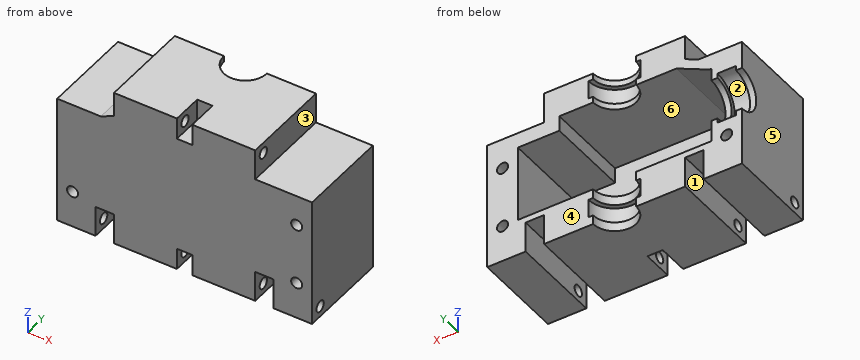
```python
from build123d import *

# Parameters (mm, degrees)
BOSS_EXTRUDE1_DEPTH  = 30
CUT_EXTRUDE2_START   = 2.5
CUT_EXTRUDE2_DEPTH   = 27.5
CUT_EXTRUDE3_START   = -2
SKETCH3_R            = 8.5
CUT_EXTRUDE3_DEPTH   = 6
CUT_EXTRUDE4_START   = -9
SKETCH4_R            = 8.5
CUT_EXTRUDE4_DEPTH   = 6
CUT_EXTRUDE6_DEPTH   = 73.981161953
SKETCH16_W           = 6
SKETCH16_H           = 30
CUT_EXTRUDE7_DEPTH   = 10
CUT_EXTRUDE8_START   = 2
SKETCH17_R           = 8.5
CUT_EXTRUDE8_DEPTH   = 6
CUT_EXTRUDE9_REACH   = 98.897
CHAMFER1_SIZE        = 2
CHAMFER1_SIZE2       = 4.289013841
CHAMFER2_SIZE        = 12.867041523
CHAMFER2_SIZE_2      = 6
SKETCH19_W           = 5
SKETCH19_H           = 7
CUT_EXTRUDE11_DEPTH  = 10
M3_CLEARANCE_HOLE1_D = 3.6
M3_CLEARANCE_HOLE2_D = 3.6


with BuildPart() as part:
    # Sketch1 → Boss-Extrude1 (new body)
    with BuildSketch(Plane(origin=(0, 0, 0), x_dir=(1, 0, 0), z_dir=(0, 1, 0))):
        Polygon((-41.5, 12), (41.5, 12), (41.5, -15), (41.5, -30), (23, -30), (23, -40), (-23, -40), (-23, -30), (-41.5, -30), (-41.5, -15), align=None)
    extrude(amount=BOSS_EXTRUDE1_DEPTH)

    # Sketch1<4> → Cut-Extrude2 (cut)
    with BuildSketch(Plane(origin=(0, 0, 0), x_dir=(1, 0, 0), z_dir=(0, 1, 0)).offset(CUT_EXTRUDE2_START)):
        Polygon((31.5, 0), (-31.5, 0), (-31.5, -10), (-31.5, -25), (-18, -25), (-18, -30), (18, -30), (18, -25), (31.5, -25), (31.5, -10), align=None)
    extrude(amount=CUT_EXTRUDE2_DEPTH, mode=Mode.SUBTRACT)

    # Sketch3 → Cut-Extrude3 (cut)
    with BuildSketch(Plane.XY.offset(40).offset(CUT_EXTRUDE3_START)):
        with Locations((0, 30)):
            Circle(SKETCH3_R)
    extrude(amount=-CUT_EXTRUDE3_DEPTH, mode=Mode.SUBTRACT)

    # Sketch4 → Cut-Extrude4 (cut)
    with BuildSketch(Plane(origin=(0, 0, -12), x_dir=(-1, 0, 0), z_dir=(0, 0, -1)).offset(CUT_EXTRUDE4_START)):
        with Locations((0, 30)):
            Circle(SKETCH4_R)
    extrude(amount=CUT_EXTRUDE4_DEPTH, mode=Mode.SUBTRACT)

    # Sketch3<4> → Cut-Extrude6 (cut, through all)
    with BuildSketch(Plane.XY.offset(40)):
        with BuildLine():
            Line((-7, 30), (7, 30))
            ThreePointArc((7, 30), (0, 37), (-7, 30))
        make_face()
        with BuildLine():
            ThreePointArc((-7, 30), (0, 23), (7, 30))
            Line((7, 30), (-7, 30))
        make_face()
        with BuildLine():
            Line((-7, 30), (7, 30))
            ThreePointArc((7, 30), (0, 37), (-7, 30))
        make_face()
        with BuildLine():
            ThreePointArc((-7, 30), (0, 23), (7, 30))
            Line((7, 30), (-7, 30))
        make_face()
    extrude(amount=-CUT_EXTRUDE6_DEPTH, mode=Mode.SUBTRACT)

    # Sketch16 → Cut-Extrude7 (cut)
    with BuildSketch(Plane(origin=(0, 0, -12), x_dir=(-1, 0, 0), z_dir=(0, 0, -1))):
        with Locations((26, 15)):
            Rectangle(SKETCH16_W, SKETCH16_H)
        with Locations((-26, 15)):
            Rectangle(SKETCH16_W, SKETCH16_H)
    extrude(amount=-CUT_EXTRUDE7_DEPTH, mode=Mode.SUBTRACT)

    # Sketch17 → Cut-Extrude8 (cut)
    with BuildSketch(Plane(origin=(-41.5, 0, 0), x_dir=(0, 0, -1), z_dir=(1, 0, 0)).offset(CUT_EXTRUDE8_START)):
        with Locations((-14, 30)):
            Circle(SKETCH17_R)
    extrude(amount=CUT_EXTRUDE8_DEPTH, mode=Mode.SUBTRACT)

    # Cut-Extrude9: up to this face of the body (flat: up to its plane)
    cut_extrude9_end = Plane(part.part.faces().sort_by_distance((-31.5, 16.25, 12.5))[0])
    # Sketch17<3> → Cut-Extrude9 (cut, up to the picked face)
    with BuildSketch(Plane(origin=(-41.5, 0, 0), x_dir=(0, 0, -1), z_dir=(1, 0, 0)), mode=Mode.PRIVATE) as cut_extrude9_sk1:
        with BuildLine():
            Line((-21, 30), (-7, 30))
            ThreePointArc((-7, 30), (-14, 37), (-21, 30))
        make_face()
    cut_extrude9_tool1 = split(extrude(cut_extrude9_sk1.sketch, amount=CUT_EXTRUDE9_REACH, mode=Mode.PRIVATE), bisect_by=cut_extrude9_end, keep=Keep.BOTH, mode=Mode.PRIVATE)
    # Sketch17<3> → Cut-Extrude9 (cut, up to the picked face)
    with BuildSketch(Plane(origin=(-41.5, 0, 0), x_dir=(0, 0, -1), z_dir=(1, 0, 0)), mode=Mode.PRIVATE) as cut_extrude9_sk2:
        with BuildLine():
            ThreePointArc((-21, 30), (-14, 23), (-7, 30))
            Line((-7, 30), (-21, 30))
        make_face()
    cut_extrude9_tool2 = split(extrude(cut_extrude9_sk2.sketch, amount=CUT_EXTRUDE9_REACH, mode=Mode.PRIVATE), bisect_by=cut_extrude9_end, keep=Keep.BOTH, mode=Mode.PRIVATE)
    # Sketch17<3> → Cut-Extrude9 (cut, up to the picked face)
    with BuildSketch(Plane(origin=(-41.5, 0, 0), x_dir=(0, 0, -1), z_dir=(1, 0, 0)), mode=Mode.PRIVATE) as cut_extrude9_sk3:
        with BuildLine():
            Line((-21, 30), (-7, 30))
            ThreePointArc((-7, 30), (-14, 37), (-21, 30))
        make_face()
    cut_extrude9_tool3 = split(extrude(cut_extrude9_sk3.sketch, amount=CUT_EXTRUDE9_REACH, mode=Mode.PRIVATE), bisect_by=cut_extrude9_end, keep=Keep.BOTH, mode=Mode.PRIVATE)
    # Sketch17<3> → Cut-Extrude9 (cut, up to the picked face)
    with BuildSketch(Plane(origin=(-41.5, 0, 0), x_dir=(0, 0, -1), z_dir=(1, 0, 0)), mode=Mode.PRIVATE) as cut_extrude9_sk4:
        with BuildLine():
            ThreePointArc((-21, 30), (-14, 23), (-7, 30))
            Line((-7, 30), (-21, 30))
        make_face()
    cut_extrude9_tool4 = split(extrude(cut_extrude9_sk4.sketch, amount=CUT_EXTRUDE9_REACH, mode=Mode.PRIVATE), bisect_by=cut_extrude9_end, keep=Keep.BOTH, mode=Mode.PRIVATE)
    add(cut_extrude9_tool1.solids().sort_by(Axis((-41.5, 32.970892, 14), (1, 0, 0)))[0], mode=Mode.SUBTRACT)
    add(cut_extrude9_tool2.solids().sort_by(Axis((-41.5, 27.029108, 14), (1, 0, 0)))[0], mode=Mode.SUBTRACT)
    add(cut_extrude9_tool3.solids().sort_by(Axis((-41.5, 32.970892, 14), (1, 0, 0)))[0], mode=Mode.SUBTRACT)
    add(cut_extrude9_tool4.solids().sort_by(Axis((-41.5, 27.029108, 14), (1, 0, 0)))[0], mode=Mode.SUBTRACT)

    # Chamfer1
    chamfer1_edges = [part.edges().sort_by_distance(p)[0] for p in [
        (-23, 15, 30),
    ]]
    chamfer1_side = [part.faces().sort_by_distance(p)[0] for p in [
        (-23, 15, 35),
    ]]
    chamfer(chamfer1_edges, length=CHAMFER1_SIZE, length2=CHAMFER1_SIZE2, reference=chamfer1_side[0])

    # Chamfer2
    # the kernel refuses this chamfer: 12.867041523, 6 mm, written as the material it takes off along each edge
    with BuildSketch(Plane(origin=(-18, 2.5, 25), x_dir=(-0.9998669641130704, 0, -0.016311164131110355), z_dir=(0, 1, 0))) as chamfer2_piece_1_section:
        Polygon((CHAMFER2_SIZE * 0.999866964118, CHAMFER2_SIZE * 0.0163111641312), (-CHAMFER2_SIZE_2 * 0.0163111641311, CHAMFER2_SIZE_2 * 0.999866964113), (0, 0), align=None)
    chamfer2_piece_1 = extrude(amount=60.838188976, mode=Mode.PRIVATE)
    chamfer2_piece_1 = split(chamfer2_piece_1, bisect_by=Plane(origin=(-22.391133218, 16.25, 30), z_dir=(0, 0, -1)), keep=Keep.TOP, mode=Mode.PRIVATE)
    add(chamfer2_piece_1, mode=Mode.SUBTRACT)

    # Sketch19 → Cut-Extrude11 (cut)
    with BuildSketch(Plane.XZ):
        with Locations((0, -8.5)):
            Rectangle(SKETCH19_W, SKETCH19_H)
        with Locations((0, 36.5)):
            Rectangle(SKETCH19_W, SKETCH19_H)
    extrude(amount=-CUT_EXTRUDE11_DEPTH, mode=Mode.SUBTRACT)

    # M3 Clearance Hole1 (through all)
    with Locations(Plane(origin=(41.5, 0, 0), x_dir=(0, 0, -1), z_dir=(1, 0, 0))):
        with Locations((8.5, 4), (-36.5, 4)):
            Hole(M3_CLEARANCE_HOLE1_D / 2)

    # M3 Clearance Hole2 (through all)
    with Locations(Plane(origin=(0, 30, 0), x_dir=(1, 0, 0), z_dir=(0, 1, 0))):
        with Locations((-36.5, 0), (36.5, 0), (36.5, -20)):
            Hole(M3_CLEARANCE_HOLE2_D / 2)


solid = part.part
```
CAD build for the part. Positions are in the model's coordinates, mm. Face numbers are marked on the shaded views. A direction names the side the tool comes from. Round coordinates to 2 decimals unless told otherwise and drop trailing zeros. Write each loop counter-clockwise with the first axis right and the second up, starting at its lowest first coordinate (ties: lowest second). Pieces come first, ordered by that corner, then holes. Notation, with made-up numbers: (88, 69.25) -> (129, 69.25) arc R23 ccw to (129, 81.25) -> close; hole circle Ø5 at (40.5, 31). An arc over 180 degrees is marked (long way). Answer in a Markdown table with one row per item. Add a question column.
Item 1: Drop flat-ended pins along their axis: pin 1 Ø3 at (x, y) = (-26, 15.5) entering from +Z; pin 2 Ø5 at (x, y) = (30, 12.5) entering from +Z; pin 3 Ø2 at (y, z) = (9, 34.5) entering from +X. Give the stop position or say it passes through.
Item 2: Drill centre lines: line 1 (X direction, y = 8, z = 20); line 2 (X direction, y = 6.5, z = -10); line 3 (Z direction, x = -1.5, y = 12.5). Where is each one in solid material? Low to high. Write a range as from..to.
Item 3: Mould opens along X. For the marked faces 4, 5 and 6 say: pulls with the +X half, pulls with the -X half, needs draft (parallel to the pull), parting line crosses it, or undercut.
Item 4: Saw through at D-D, the plane y = 4. Count the separate pieces of the cut face and the enclosed holes in it, then the cut area to 3 significant figures.
Item 5: Saw through at A-A, the plane z = 36.5. Write the cut outline in (x, y).
Item 6: Saw through at C-C, the plane y = 15. Write the cut outline in (x, z).
Item 7: Saw through at B-B, the plane x = 36.5. Write the cut outline in (y, z).
Item 8: Which spindle directions (+Z, -Z, +X, -X, +Y, -Y) get a long thin tool onto all of the face, cutting with end or side? Do the marked faces 1, 2 and 3. Say none if no direction does.
Findings below:
| question | item | result |
|---|---|---|
| 1 | pin 1 | stops at z = 31.3 |
| 1 | pin 2 | stops at z = 30 |
| 1 | pin 3 | stops at x = 23 |
| 2 | line 1 | x = -41.5..-31.5, 31.5..34.7, 38.3..41.5 |
| 2 | line 2 | x = -41.5..-29, -23..-2.5, 2.5..23, 29..41.5 |
| 2 | line 3 | z = -12..0, 30..40 |
| 3 | face 4 | needs draft |
| 3 | face 5 | pulls with the -X half |
| 3 | face 6 | undercut |
| 4 | separate pieces | 7 |
| 4 | enclosed holes | 4 |
| 4 | area | 1,550 mm^2 |
| 5 | outline | (-23, 0) -> (-2.5, 0) -> (-2.5, 2.2) -> (-23, 2.2) -> close; (-23, 5.8) -> (-2.5, 5.8) -> (-2.5, 10) -> (2.5, 10) -> (2.5, 5.8) -> (23, 5.8) -> (23, 30) -> (8.5, 30) arc R8.5 cw to (-8.5, 30) -> (-23, 30) -> close; (2.5, 0) -> (23, 0) -> (23, 2.2) -> (2.5, 2.2) -> close |
| 6 | outline | (-41.5, -12) -> (-29, -12) -> (-29, -2) -> (-23, -2) -> (-23, -12) -> (23, -12) -> (23, -2) -> (29, -2) -> (29, -12) -> (41.5, -12) -> (41.5, 30) -> (23, 30) -> (23, 40) -> (-23, 40) -> (-23, 32) -> (-27.29, 30) -> (-41.5, 30) -> close; hole circle Ø3.6 at (-36.5, 0); hole (-31.5, 0) -> (31.5, 0) -> (31.5, 25) -> (18, 25) -> (18, 30) -> (-20.14, 30) -> (-30.87, 25) -> (-31.5, 25) -> close; hole circle Ø3.6 at (36.5, 0); hole circle Ø3.6 at (36.5, 20) |
| 7 | outline | (0, -12) -> (30, -12) -> (30, -1.8) -> (0, -1.8) -> close; (0, 1.8) -> (30, 1.8) -> (30, 18.2) -> (0, 18.2) -> close; (0, 21.8) -> (30, 21.8) -> (30, 30) -> (0, 30) -> close; hole circle Ø3.6 at (4, -8.5) |
| 8 | face 1 | -Z, +Y, -Y |
| 8 | face 2 | +Y |
| 8 | face 3 | +Z, +X, +Y, -Y |
